CAD build for the part. Positions are in the model's coordinates, mm. Round coordinates to 2 decimals unless told otherwise and drop trailing zeros. Order: outer loops, then holes, each group sorted by start corner. A loop starts at its lowest first (then second) coordinate and runs counter-clockwise, first axis right, second up. Notation, with made-up numbers: (72, 13) -> (127, 13) arc R21 cw to (127, 19) -> close; hole circle Ø1 at (-39, 64). An arc over 180 degrees is marked (long way). Answer as CSV lines item,"result". Start each with the question number.
from build123d import *

# Parameters (mm, degrees)
F1_DEPTH      = 825
F3_DEPTH      = 20.001
F3_DEPTH_BACK = 20.001


# Not quite as in the source:
# - a pattern or mirror of a feature is missing from the dataset's text; its kind, count and spacing are read off the source's solid


with BuildPart() as f1:
    # F0 (on Top) → F1 (new body, symmetric)
    with BuildSketch(Plane.XY):
        with BuildLine():
            Line((17, 20), (-17, 20))
            ThreePointArc((-17, 20), (-19.1213203436, 19.1213203436), (-20, 17))
            Line((-20, 17), (-20, -17))
            ThreePointArc((-20, -17), (-19.1213203436, -19.1213203436), (-17, -20))
            Line((-17, -20), (17, -20))
            ThreePointArc((17, -20), (19.1213203436, -19.1213203436), (20, -17))
            Line((20, -17), (20, 17))
            ThreePointArc((20, 17), (19.1213203436, 19.1213203436), (17, 20))
        make_face()
        with BuildLine():
            ThreePointArc((-18, 17), (-17.7071067812, 17.7071067812), (-17, 18))
            Line((-17, 18), (17, 18))
            ThreePointArc((17, 18), (17.7071067812, 17.7071067812), (18, 17))
            Line((18, 17), (18, -17))
            ThreePointArc((18, -17), (17.7071067812, -17.7071067812), (17, -18))
            Line((17, -18), (-17, -18))
            ThreePointArc((-17, -18), (-17.7071067812, -17.7071067812), (-18, -17))
            Line((-18, -17), (-18, 17))
        make_face(mode=Mode.SUBTRACT)
    extrude(amount=F1_DEPTH, both=True)

    # F2 (on Front) → F3 (cut, two sides)
    with BuildSketch(Plane.XZ) as f3_sk:
        Polygon((20, 825), (-20, 825), (-20, 785), align=None)
    f3 = extrude(amount=-F3_DEPTH, mode=Mode.SUBTRACT) + extrude(f3_sk.sketch, amount=F3_DEPTH_BACK, mode=Mode.SUBTRACT)

    # F3_copies: F3 across plane
    add(f3.mirror(Plane(origin=(0, 0, 0), x_dir=(-1, 0, 0), z_dir=(0, 0, -1))), mode=Mode.SUBTRACT)


solid = f1.part
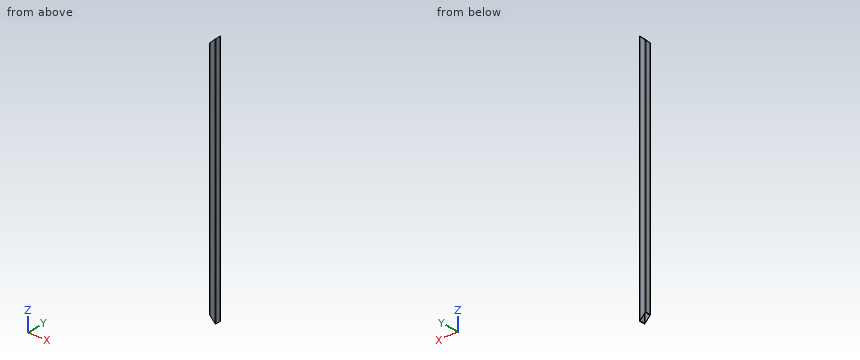
Item 1: Band-saw the part on B-B, the plane x = 7.5. Give the cut face in (y, z), and give its area (3 significant figures).
Item 2: Probe line 1 (Y direction, x = -2, z = -538.5). List the from-to ranges inside material, lowest first.
Item 3: Band-saw the part on C-C, the plane z = -330.5. Give the cut face in (x, y).
Item 4: Pin check, flat tip, straight feed: pin 1 (10 mm diameter, centred on x = 11.5, y = 11, fed in from -Z). Stop position of the tip, or through.
Item 5: Band-saw the part on A-A, the plane y = 1. Give the cut face in (x, z), and give its area (3 significant figures).
Values:
1,outline,"(-20, -812.5) -> (-18, -812.5) -> (-18, 812.5) -> (-20, 812.5) -> close; (18, -812.5) -> (20, -812.5) -> (20, 812.5) -> (18, 812.5) -> close"
1,area,"6,500 mm²"
2,line 1,"-20 to -18, 18 to 20"
3,outline,"(-20, -17) arc R3 ccw to (-17, -20) -> (17, -20) arc R3 ccw to (20, -17) -> (20, 17) arc R3 ccw to (17, 20) -> (-17, 20) arc R3 ccw to (-20, 17) -> close; hole (-18, -17) arc R1 ccw to (-17, -18) -> (17, -18) arc R1 ccw to (18, -17) -> (18, 17) arc R1 ccw to (17, 18) -> (-17, 18) arc R1 ccw to (-18, 17) -> close"
4,pin 1,"through"
5,outline,"(-20, -785) -> (-18, -787) -> (-18, 787) -> (-20, 785) -> close; (18, -823) -> (20, -825) -> (20, 825) -> (18, 823) -> close"
5,area,"6,440 mm²"
